from build123d import *

# Parameters (mm, degrees)
SKETCH_W        = 20
SKETCH_H        = 16
PAD_DEPTH       = 6.5
POCKET_DEPTH    = 1.75
POCKET002_DEPTH = 16.001
FILLET_R        = 0.5
SKETCH004_R     = 1.1
POCKET003_DEPTH = 8
SKETCH005_R     = 1.35
POCKET004_DEPTH = 7
SKETCH006_W     = 9
SKETCH006_H     = 9
POCKET005_DEPTH = 3
CHAMFER_1_ANGLE = 60
CHAMFER_1_SIZE  = 1.5
CHAMFER_2_ANGLE = 60
CHAMFER_2_SIZE  = 1.5
FILLET001_R     = 0.5
FILLET002_R     = 0.5
FILLET003_R     = 1
FILLET004_R     = 0.5
SKETCH007_W     = 2
SKETCH007_H     = 5
PAD001_DEPTH    = 0.2


with BuildPart() as part:
    # Sketch (on XY_Plane of Origin) → Pad (new body, symmetric)
    with BuildSketch(Plane.XY):
        Rectangle(SKETCH_W, SKETCH_H)
    extrude(amount=PAD_DEPTH, both=True)

    # Sketch001 → Pocket (cut, symmetric)
    with BuildSketch(Plane.XY):
        Polygon((-7.287187, 8), (-3, -8), (7, -8), (7, 8), align=None)
    extrude(amount=POCKET_DEPTH, both=True, mode=Mode.SUBTRACT)

    # Sketch003 (on Face1 of Pocket) → Pocket002 (cut, through all)
    with BuildSketch(Plane.XZ.offset(8)):
        with BuildLine():
            ThreePointArc((6.646447, -2.103553), (7.353553, -2.103553), (7.353553, -1.396447))
            Line((7.353553, -1.396447), (6.646447, -0.68934))
            ThreePointArc((6.646447, -0.68934), (5.93934, -0.68934), (5.93934, -1.396447))
            Line((6.646447, -2.103553), (5.93934, -1.396447))
        make_face()
        with BuildLine():
            ThreePointArc((7.353553, 1.396447), (7.353553, 2.103553), (6.646447, 2.103553))
            Line((6.646447, 2.103553), (5.93934, 1.396447))
            ThreePointArc((5.93934, 1.396447), (5.93934, 0.68934), (6.646447, 0.68934))
            Line((7.353553, 1.396447), (6.646447, 0.68934))
        make_face()
    extrude(amount=-POCKET002_DEPTH, mode=Mode.SUBTRACT)

    # Fillet
    fillet_edges = [part.edges().sort_by_distance(p)[0] for p in [
        (6.292893, 0, -1.75),
        (6.292893, 0, 1.75),
        (7, 0, -1.042893),
        (7, 0, 1.042893),
    ]]
    fillet(fillet_edges, radius=FILLET_R)

    # Sketch004 (on XY_Plane of Origin) → Pocket003 (cut, symmetric)
    with BuildSketch(Plane.XY):
        with Locations((2, 4.5)):
            Circle(SKETCH004_R)
        with Locations((2, -4.5)):
            Circle(SKETCH004_R)
    extrude(amount=POCKET003_DEPTH, both=True, mode=Mode.SUBTRACT)

    # Sketch005 (on Face16 of Pocket003) → Pocket004 (cut)
    with BuildSketch(Plane(origin=(-10, 0, 0), x_dir=(0, -1, 0), z_dir=(-1, 0, 0))):
        Circle(SKETCH005_R)
    extrude(amount=-POCKET004_DEPTH, mode=Mode.SUBTRACT)

    # Sketch006 (on Face19 of Pocket004) → Pocket005 (cut)
    with BuildSketch(Plane.YZ.offset(10)):
        Rectangle(SKETCH006_W, SKETCH006_H)
    extrude(amount=-POCKET005_DEPTH, mode=Mode.SUBTRACT)

    # Chamfer 1
    chamfer_1_edges = [part.edges().sort_by_distance(p)[0] for p in [
        (8.5, 4.5, -4.5),
        (8.5, 4.5, 4.5),
    ]]
    chamfer_1_side = part.faces().sort_by_distance((8.542167, 4.5, 0))[0]
    chamfer(chamfer_1_edges, length=CHAMFER_1_SIZE, angle=CHAMFER_1_ANGLE, reference=chamfer_1_side)

    # Chamfer 2
    chamfer_2_edges = [part.edges().sort_by_distance(p)[0] for p in [
        (8.5, -4.5, -4.5),
        (8.5, -4.5, 4.5),
    ]]
    chamfer_2_side = part.faces().sort_by_distance((8.542167, -4.5, 0))[0]
    chamfer(chamfer_2_edges, length=CHAMFER_2_SIZE, angle=CHAMFER_2_ANGLE, reference=chamfer_2_side)

    # Fillet001
    fillet001_edges = [part.edges().sort_by_distance(p)[0] for p in [
        (7, 0, 2.25),
        (7, 0, -2.25),
    ]]
    fillet(fillet001_edges, radius=FILLET001_R)

    # Fillet002
    fillet002_edges = [part.edges().sort_by_distance(p)[0] for p in [
        (7, -3.200962, -3.75),
        (7, 0, -4.5),
        (7, 3.200962, -3.75),
        (7, -3.200962, 3.75),
        (7, 0, 4.5),
        (7, 3.200962, 3.75),
    ]]
    fillet(fillet002_edges, radius=FILLET002_R)

    # Fillet003
    fillet003_edges = [part.edges().sort_by_distance(p)[0] for p in [
        (10, 0, 6.5),
        (-10, 0, 6.5),
        (-10, 0, -6.5),
        (10, 0, -6.5),
    ]]
    fillet(fillet003_edges, radius=FILLET003_R)

    # Fillet004
    fillet004_edges = [part.edges().sort_by_distance(p)[0] for p in [
        (10, -3.200962, -3.75),
        (10, 0, -4.5),
        (10, 3.200962, -3.75),
        (10, 3.200962, 3.75),
        (10, 0, 4.5),
        (10, -3.200962, 3.75),
    ]]
    fillet(fillet004_edges, radius=FILLET004_R)

    # Sketch007 (on Face8 of Fillet004) → Pad001 (join)
    with BuildSketch(Plane.XZ.offset(-4.5)):
        with Locations((8, 0)):
            Rectangle(SKETCH007_W, SKETCH007_H)
    extrude(amount=-PAD001_DEPTH)


solid = part.part
Verification items for the finished model (mm, model axes). A direction names the side the tool comes from. Round coordinates to 2 decimals unless told otherwise and drop trailing zeros. Loops run counter-clockwise (first coordinate to the right, second up) from the corner with the lowest first, then second, coordinate; pieces in that order, holes last. Notation, with made-up numbers: M -24.75,73.25 L 4.25,73.25 A24 ccw 4.25,94.25 Z; hole C 13.25,21 d9. An arc over 180 degrees is marked long. Write each question's results on one line, items separated by ' | '.
1) Section check D-D on z = 0. Record the boundary of the cut face in (x, y), then the cut area to 3 significant figures.
Checks:
outline: M -10,-8 L -3,-8 L -4.78,-1.35 L -10,-1.35 Z; M -10,1.35 L -5.51,1.35 L -7.29,8 L -10,8 Z; M 7,-8 L 10,-8 L 10,-4.5 L 7,-4.5 Z; M 7,4.5 L 10,4.5 L 10,8 L 7,8 Z | area: 85.6 mm2
2) Scan lines: L1, parallel to Y at x = 2, z = 4; L2, parallel to Y at x = 7.75, z = -0.5; L3, parallel to Z at x = 3, y = 0.75. Record each from-to range of solid material in increasing order. Write a range as from..to.
Checks:
L1: y = -8..-5.6, -3.4..3.4, 5.6..8 | L2: y = -8..-4.5, 4.5..8 | L3: z = -6.5..-1.75, 1.75..6.5
3) Section check C-C on x = 2. Record the boundary of the cut face in (y, z).
Checks:
outline: M -8,-6.5 L -5.6,-6.5 L -5.6,-1.75 L -8,-1.75 Z; M -8,1.75 L -5.6,1.75 L -5.6,6.5 L -8,6.5 Z; M -3.4,-6.5 L 3.4,-6.5 L 3.4,-1.75 L -3.4,-1.75 Z; M -3.4,1.75 L 3.4,1.75 L 3.4,6.5 L -3.4,6.5 Z; M 5.6,-6.5 L 8,-6.5 L 8,-1.75 L 5.6,-1.75 Z; M 5.6,1.75 L 8,1.75 L 8,6.5 L 5.6,6.5 Z
4) Mould release check, pull along Z, two halves, no side actions. Record for faces 1 (the cylindrical face through (9.857, 3.199, -3.925)), 2 (the cylindrical face through (9.715, 0.112, 6.199)), 3 (the cylindrical face through (2.59, -3.57, 4.16)): released by +Z, released by -Z, zero draft, split by the parting line, or undercut.
Checks:
face 1: undercut | face 2: released by +Z | face 3: zero draft
5) Section check B-B on z = 5.25. Record the boundary of the cut face in (x, y).
Checks:
outline: M -10,-8 L 10,-8 L 10,8 L -10,8 Z; hole C 2,-4.5 d2.2; hole C 2,4.5 d2.2
6) Gauge pin test, flat end, axial feed: P1, Ø5, axis at y = -1.5, z = 0.5, coming from the +X side. Record the tip position at first contact, or that the pin passes through.
Checks:
P1: stops at x = 7
7) Access from +Z, -Z, +X, -X, +Y, -Y to the whole of each face (thin tool, end or side, straight path). Record for faces 4 (the flat face through (7, 0, -3)), 5 (the flat face through (1, 0, 1.75)), 6 (the flat face through (7, 6, 0)), 7 (the cylindrical face through (-7.427, -1.288, 0.406)).
Checks:
face 4: +X | face 5: +Y | face 6: +Y, -Y | face 7: +X, -X
